Job drawing, mm, ordinate dimensions from the low corner. One solid piece. A direction names the side the tool comes from. Coordinates: 2 decimals unless noted, no trailing zeros. Write each loop counter-clockwise with the first axis right and the second up, starting at its lowest first coordinate (ties: lowest second). Pieces come first, ordered by that corner, then holes. Notation, with made-up numbers: (65, -15) -> (76, -15) arc R32 cw to (76, 24) -> close; hole circle Ø3 at (52, 12). An arc over 180 degrees is marked (long way). Answer as a JSON object with one key per item and string values. Group by question number.
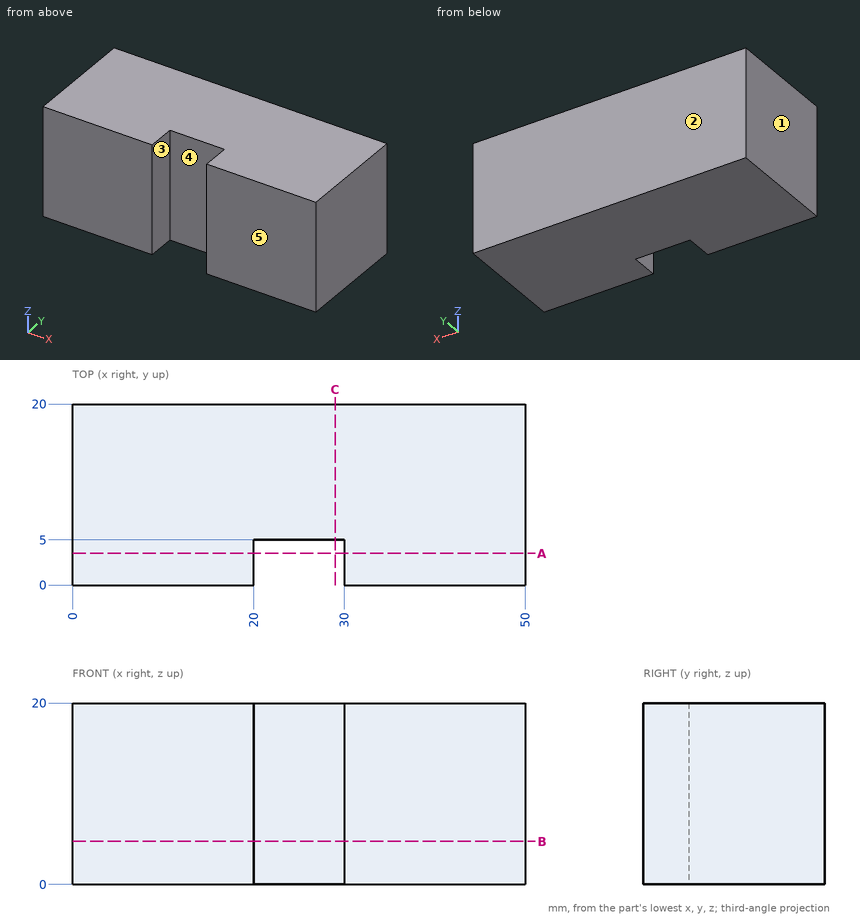
(1) 3-axis set-ups, long thin cutter, end or side, ignore diameter. For the marked faces 4 and 5: which of +Z, -Z, +X, -X, +Y, -Y reach the whole face in a straight line?
(2) Pin check, flat tip, straight feed: pin 1 (3 mm diameter, centred on x = 8.5, z = 9.5, fed in from -Y). Stop position of the tip, or through.
(3) Pull direction X, two halves, no side cores. Call the marked faces 1, 2 and 3: released by +X, released by -X, zero draft, split by the parting line, or undercut.
(4) Cut at A-A on y = 3.5. List the corners of the cut face in (x, z), plus the area to 3 significant figures.
(5) Wall check: probe 1 along X at (y, z) = (3.5, 2); probe 2 along Y at (x, z) = (24.5, 8.5). Give the ranges that are in metal, low to high.
(6) Cut at B-B on z = 4.75. List the corners of the cut face in (x, y).
(7) Cut at C-C on x = 29. List the corners of the cut face in (y, z), plus the area to 3 significant figures.
Results found:
{
 "1": {"face 4": "+Z, -Z, -Y", "face 5": "+Z, -Z, +X, -X, -Y"},
 "2": {"pin 1": "stops at y = 0"},
 "3": {"face 1": "released by -X", "face 2": "zero draft", "face 3": "undercut"},
 "4": {"outline": "(0, 0) -> (20, 0) -> (20, 20) -> (0, 20) -> close; (30, 0) -> (50, 0) -> (50, 20) -> (30, 20) -> close", "area": "800 mm²"},
 "5": {"probe 1": "x = 0 to 20, 30 to 50", "probe 2": "y = 5 to 20"},
 "6": {"outline": "(0, 0) -> (20, 0) -> (20, 5) -> (30, 5) -> (30, 0) -> (50, 0) -> (50, 20) -> (0, 20) -> close"},
 "7": {"outline": "(5, 0) -> (20, 0) -> (20, 20) -> (5, 20) -> close", "area": "300 mm²"}
}
